Drawing for the job (mm, zero at the part's lowest x, y, z). A direction names the side the tool comes from. Coordinates: 2 decimals unless noted, no trailing zeros. Loops run counter-clockwise (first coordinate to the right, second up) from the corner with the lowest first, then second, coordinate; pieces in that order, holes last. Notation, with made-up numbers: (89.5, 53.5) - (129.5, 53.5) arc R32 ccw to (129.5, 89.5) - close; hole circle Ø5 at (46.25, -20). An arc over 180 degrees is marked (long way). One line per item, written item: value.
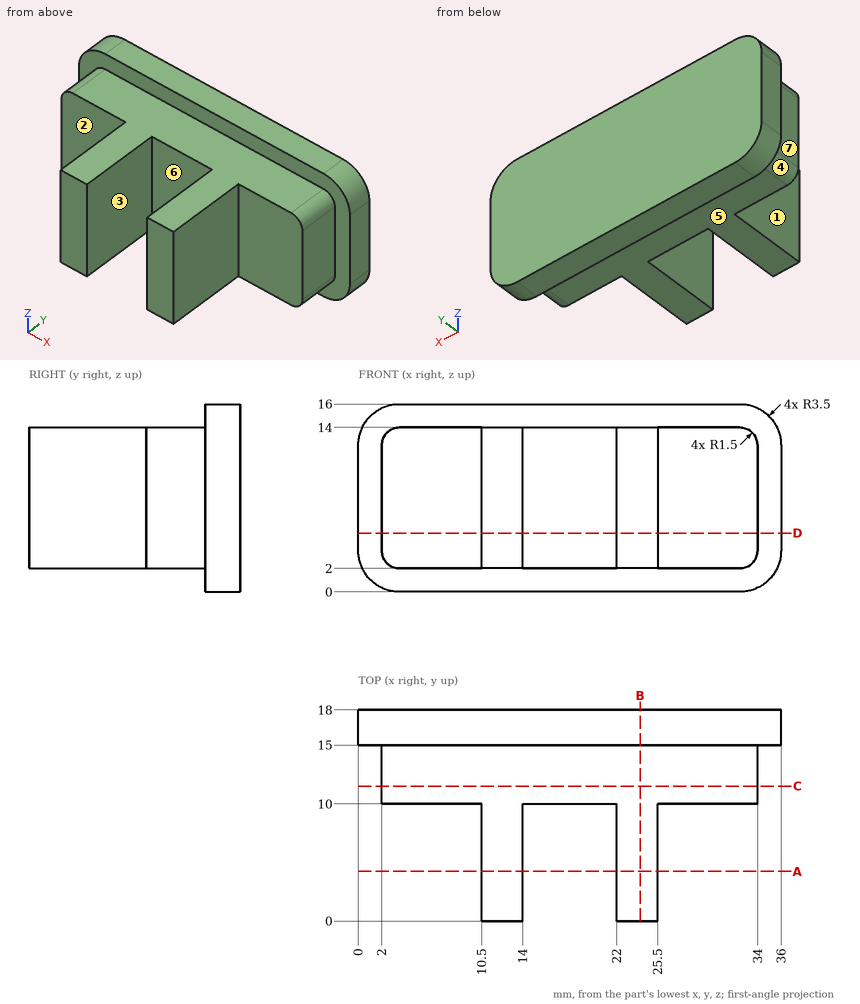
Item 1: Cut at B-B, the plane x = 24. Write the cut outline in (y, z), then the cut area to 3 significant figures.
Check result:
outline: (0, 2) - (15, 2) - (15, 0) - (18, 0) - (18, 16) - (15, 16) - (15, 14) - (0, 14) - close
area: 228 mm^2
Item 2: Tool access for the marked faces 4, 5, 6 and 7: list every direction of +Z, -Z, +X, -X, +Y, -Y with a clear straight run to the whole face (end or side of a thin tool).
Check result:
face 4: -Z, -X, -Y
face 5: -Z, +X, -X, -Y
face 6: +Z, -Z, -Y
face 7: +Z, -Z, -X, -Y
Item 3: Cut at C-C, the plane y = 11.5. Write the cut outline in (x, z).
Check result:
outline: (2, 3.5) arc R1.5 ccw to (3.5, 2) - (32.5, 2) arc R1.5 ccw to (34, 3.5) - (34, 12.5) arc R1.5 ccw to (32.5, 14) - (3.5, 14) arc R1.5 ccw to (2, 12.5) - close
Item 4: Cut at A-A, the plane y = 4.25. Write the cut outline in (x, z), then the cut area to 3 significant figures.
Check result:
outline: (10.5, 2) - (14, 2) - (14, 14) - (10.5, 14) - close; (22, 2) - (25.5, 2) - (25.5, 14) - (22, 14) - close
area: 84.0 mm^2
Item 5: Cut at D-D, the plane z = 5. Write the cut outline in (x, y).
Check result:
outline: (0, 15) - (2, 15) - (2, 10) - (10.5, 10) - (10.5, 0) - (14, 0) - (14, 10) - (22, 10) - (22, 0) - (25.5, 0) - (25.5, 10) - (34, 10) - (34, 15) - (36, 15) - (36, 18) - (0, 18) - close
Item 6: Drop flat-ended pins along their axis: P1, Ø4, axis at y = 2.5, z = 4, coming from the -X side; P2, Ø7, axis at x = 7.5, z = 9.5, coming from the -Y side; P3, Ø5, axis at y = 6.5, z = 10, coming from the +X side; P4, Ø7.5, axis at x = 22.5, y = 8.5, coming from the +Z side. Give the stop position or say it passes through.
Check result:
P1: stops at x = 10.5
P2: stops at y = 0
P3: stops at x = 25.5
P4: stops at z = 14
Item 7: Pull direction X, two halves, no side cores. Call the marked faces 1, 2 and 3: released by +X, released by -X, zero draft, split by the parting line, or undercut.
Check result:
face 1: released by -X
face 2: zero draft
face 3: undercut
Item 8: Probe probe 1 along X at (y, z) = (3, 3.25); probe 2 along X at (y, z) = (11.5, 8.25); probe 3 along Z at (x, y) = (29.5, 11.75). List the from-to ranges inside material, lowest first. Write a range as from..to.
Check result:
probe 1: x = 10.5..14, 22..25.5
probe 2: x = 2..34
probe 3: z = 2..14
